Source: CAD feature listing. Evaluate the final solid. Frame: model axes, mm. Face numbers are marked on the shaded views. A direction names the side the tool comes from. Give positions to 0.01 mm unless a question says otherwise; leave off trailing zeros. Write each loop counter-clockwise with the first axis right and the second up, starting at its lowest first coordinate (ties: lowest second). Pieces come first, ordered by that corner, then holes.
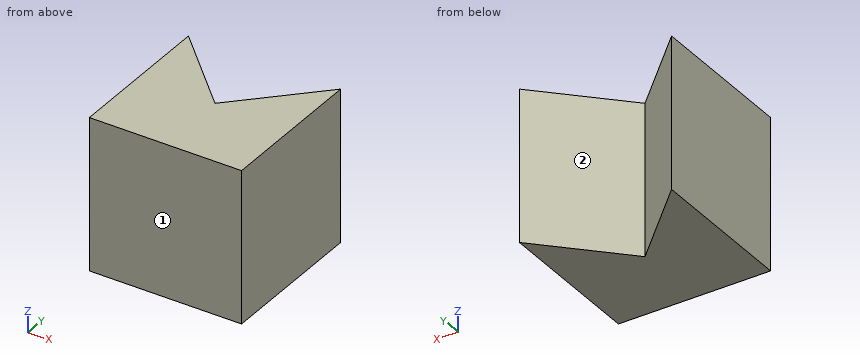
Autodesk Inventor part; units mm, degrees
ref_plane "YZ Plane" through (0, 0, 0) normal (1, 0, 0) x (0, 1, 0)
ref_plane "XZ Plane" through (0, 0, 0) normal (0, 1, 0) x (-1, 0, 0)
ref_plane "XY Plane" through (0, 0, 0) normal (0, 0, 1) x (1, 0, 0)
sketch "Sketch1" plane through (0, 0, 0) normal (0, 1, 0) x (-1, 0, 0)
  line L0 (0, 0) -> (25.4, 0)
  line L1 (25.4, 0) -> (25.4, -25.4)
  line L2 (25.4, -25.4) -> (0, -25.4)
  line L3 (0, -25.4) -> (0, 0)
  dimension "d0" = 25.4
  dimension "d1" = 25.4
extrude "Extrusion1" add sketch "Sketch1" along normal blind 25.4
sketch "Sketch2" plane through (0, 0, -25.4) normal (0, 0, -1) x (-1, 0, 0)
  line L0 (25.4, 25.4) -> (0, 25.4)
  line L1 (12.7, 12.7) -> (0, 25.4)
  line L2 (0, 25.4) -> (25.4, 25.4)
  line L3 (25.4, 25.4) -> (12.7, 12.7)
  point P0 (0, 0)
extrude "Extrusion2" cut sketch "Sketch2" against normal blind 25.4
properties part number "2 color test pt1"
1. Section query C-C (x = -2). Return loops of the section in (y, z).
2. Pin query (flat end, axial travel): P1, Ø1, axis at x = -10, z = -7, coming from the +Y side; P2, Ø6, axis at x = -6, z = -6, coming from the +Y side; P3, Ø1.5, axis at x = -19, z = -8.5, coming from the +Y side. Return the tip coordinate at first contact, or that it passes through.
3. Section query D-D (x = -6.75). Return loops of the section in (y, z), plus the area to 3 significant figures.
4. Section query B-B (z = -14). Return loops of the section in (x, y), plus the area to 3 significant figures.
5. Section query A-A (y = 20.5). Return loops of the section in (x, z), plus the area to 3 significant figures.
6. Access query for the marked faces 1 and 2. Directions: +Z, -Z, +X, -X, +Y, -Y. A direction counts if a zero-diameter tool reaches every point of the face in a straight line with its end or side. Return the directions, or none.
7. Line query: probe 1 along X at (y, z) = (21.25, -17.75); probe 2 along X at (y, z) = (14, -14.25); probe 3 along Y at (x, z) = (-6, -6). Output: solid intervals per line, ascending.
The answers:
1. outline: (0, -25.4) - (23.4, -25.4) - (23.4, 0) - (0, 0) - close
2. P1: stops at y = 15.9
2. P2: stops at y = 22.4
2. P3: stops at y = 19.75
3. outline: (0, -25.4) - (18.65, -25.4) - (18.65, 0) - (0, 0) - close
3. area: 474 mm2
4. outline: (-25.4, 0) - (0, 0) - (0, 25.4) - (-12.7, 12.7) - (-25.4, 25.4) - close
4. area: 484 mm2
5. outline: (-25.4, -25.4) - (-20.5, -25.4) - (-20.5, 0) - (-25.4, 0) - close; (-4.9, -25.4) - (0, -25.4) - (0, 0) - (-4.9, 0) - close
5. area: 249 mm2
6. face 1: +Z, -Z, +X, -X, -Y
6. face 2: +Z, -Z, +Y
7. probe 1: x = -25.4 to -21.25, -4.15 to 0
7. probe 2: x = -25.4 to -14, -11.4 to 0
7. probe 3: y = 0 to 19.4
